CAD build for the part. Positions are in the model's coordinates, mm. A direction names the side the tool comes from. Give positions to 0.01 mm unless a question says otherwise; leave off trailing zeros. Loops run counter-clockwise (first coordinate to the right, second up) from the corner with the lowest first, then second, coordinate; pieces in that order, holes last. Notation, with made-up numbers: M -39,-5 L -33,-5 A17 ccw -33,19 Z; hole C -26,82.25 d10. An arc over 180 degrees is marked long. One line per question, with ' | ' between items.
```python
from build123d import *

# Parameters (mm, degrees)
SKETCH1_W           = 5
SKETCH1_H           = 5
BOSS_EXTRUDE1_DEPTH = 5
CUT_EXTRUDE1_DEPTH  = 2
CUT_EXTRUDE7_DEPTH  = 1
SKETCH6_W           = 2
SKETCH6_H           = 4
CUT_EXTRUDE13_DEPTH = 1
CUT_EXTRUDE14_DEPTH = 2
CUT_EXTRUDE16_DEPTH = 3
CUT_EXTRUDE17_DEPTH = 2


with BuildPart() as part:
    # Sketch1 → Boss-Extrude1 (new body)
    with BuildSketch(Plane.XY):
        Rectangle(SKETCH1_W, SKETCH1_H)
    extrude(amount=BOSS_EXTRUDE1_DEPTH)

    # Sketch2 → Cut-Extrude1 (cut)
    with BuildSketch(Plane(origin=(0, 2.5, 0), x_dir=(1, 0, 0), z_dir=(0, 1, 0))):
        Polygon((-2.5, -5), (0.5, -5), (0.5, -2), (-1.5, -2), (-1.5, -4), (-2.5, -4), align=None)
    extrude(amount=-CUT_EXTRUDE1_DEPTH, mode=Mode.SUBTRACT)

    # Sketch3 → Cut-Extrude7 (cut)
    with BuildSketch(Plane.ZY.offset(2.5)):
        Polygon((4, 0.5), (2, 2.5), (4, 2.5), align=None)
    extrude(amount=-CUT_EXTRUDE7_DEPTH, mode=Mode.SUBTRACT)

    # Sketch6 → Cut-Extrude13 (cut)
    with BuildSketch(Plane.XY.offset(5)):
        with Locations((1.5, 0.5)):
            Rectangle(SKETCH6_W, SKETCH6_H)
    extrude(amount=-CUT_EXTRUDE13_DEPTH, mode=Mode.SUBTRACT)

    # Sketch7 → Cut-Extrude14 (cut)
    with BuildSketch(Plane(origin=(2.5, 0, 0), x_dir=(0, 0, -1), z_dir=(1, 0, 0))):
        Polygon((-4, 2.5), (-2, 2.5), (-2, 0.5), (-4, -1.5), align=None)
    extrude(amount=-CUT_EXTRUDE14_DEPTH, mode=Mode.SUBTRACT)

    # Sketch8 → Cut-Extrude16 (cut, through all)
    with BuildSketch(Plane.XY.offset(2)):
        Polygon((2.5, 2.5), (1.5, 2.5), (2.5, 0.5), align=None)
    extrude(amount=-CUT_EXTRUDE16_DEPTH, mode=Mode.SUBTRACT)

    # Sketch10 → Cut-Extrude17 (cut)
    with BuildSketch(Plane(origin=(0, 2.5, 0), x_dir=(1, 0, 0), z_dir=(0, 1, 0))):
        Polygon((2.5, -2), (2.5, -1), (1.5, -1), (0.5, -2), align=None)
    extrude(amount=-CUT_EXTRUDE17_DEPTH, mode=Mode.SUBTRACT)


solid = part.part
```
Item 1: 3-axis set-ups, long thin cutter, end or side, ignore diameter. For faces 1 (the flat face through (1.7, 0.5, 1.5)), 2 (the flat face through (-2, 1.5, 3)): which of +Z, -Z, +X, -X, +Y, -Y reach the whole face in a straight line?
Conclusion:
face 1: +Z, +X, +Y | face 2: +Z, +X, -X, +Y
Item 2: Saw through at B-B on x = 0.8. Give the cut face in (y, z).
Conclusion:
outline: M -2.5,0 L 2.5,0 L 2.5,1.7 L 0.5,1.7 L 0.5,2 L -1.5,4 L -1.5,5 L -2.5,5 Z
Item 3: Drill centre lines: line 1 along Y through (x, z) = (-1.15, 2.5); line 2 along Y through (x, z) = (0.8, 4.4). Where is each one in solid material? Low to high. Write a range as [from, to].
Conclusion:
line 1: [-2.5, 0.5] | line 2: [-2.5, -1.5]
Item 4: Drop flat-ended pins along their axis: P1, Ø1.6, axis at y = 1.5, z = 2.5, coming from the +X side; P2, Ø1.5, axis at x = -1.5, y = 1.5, coming from the +Z side. Give the stop position or say it passes through.
Conclusion:
P1: x = 0.8 | P2: z = 3.75
Item 5: Saw through at A-A on y = 2.1. Give the cut face in (x, z), and give its area (3 significant figures).
Conclusion:
outline: M -2.5,0 L 1.7,0 L 1.7,1 L 1.5,1 L 0.5,2 L -1.5,2 L -1.5,2.4 L -2.5,2.4 Z | area: 8.10 mm²
Item 6: Saw through at D-D on x = -1.8. Give the cut face in (y, z).
Conclusion:
outline: M -2.5,0 L 2.5,0 L 2.5,2 L 0.5,4 L 0.5,5 L -2.5,5 Z
Item 7: Saw through at C-C on z = 4.3. Give the cut face in (x, y), and give its area (3 significant figures).
Conclusion:
outline: M -2.5,-2.5 L 2.5,-2.5 L 2.5,-1.5 L 0.5,-1.5 L 0.5,0.5 L -2.5,0.5 Z | area: 11.0 mm²
